Could you check a few things on this model? Use its own coordinates, in mm. A direction names the side the tool comes from. Round coordinates to 2 decimals unless told otherwise and drop trailing zeros. Order: outer loops, then holes, each group sorted by start corner. A loop starts at its lowest first (then second) coordinate and runs counter-clockwise, first axis right, second up. Notation, with made-up numbers: (18, 17) - (36, 17) arc R16 cw to (36, 25) - close; hole circle Ø3 at (50, 25). An arc over 180 degrees is marked (long way). Use one line per item in the form item = value.
from build123d import *

# Parameters (mm, degrees)
F1_DEPTH = 496
F2_R     = 6
F3_DEPTH = 40
F5_W     = 650
F5_H     = 10
F6_DEPTH = 10
F7_W     = 10
F7_H     = 476
F8_DEPTH = 10


# Not quite as in the source:
# - a pattern or mirror of a feature is missing from the dataset's text; its kind, count and spacing are read off the source's solid


with BuildPart() as f1:
    # F0 (on Front) → F1 (new body)
    with BuildSketch(Plane.XZ):
        Polygon((374.2424272732, 0), (-325.7575727268, 0), (-325.7575727268, -40), (-285.7575727268, -40), (-285.7575727268, -20), (344.2424272732, -20), (344.2424272732, -40), (374.2424272732, -40), align=None)
    extrude(amount=F1_DEPTH)

    # F2 (on face) → F3 (join)
    with BuildSketch(Plane(origin=(0, 0, 0), x_dir=(-1, 0, 0), z_dir=(0, 1, 0))):
        with Locations((-359.2424272732, -20)):
            Circle(F2_R)
        with Locations((305.7575727268, -20)):
            Circle(F2_R)
    f3 = extrude(amount=F3_DEPTH)

    # F3_copies: F3 across plane
    add(f3.mirror(Plane(origin=(0, -248, 0), x_dir=(0, 0, -1), z_dir=(0, -1, 0))))

    # F5 (on face) → F6 (cut)
    with BuildSketch(Plane(origin=(0, 0, 0), x_dir=(-1, 0, 0), z_dir=(0, 1, 0))):
        with Locations((-39.2424272732, -5)):
            Rectangle(F5_W, F5_H)
    f6 = extrude(amount=-F6_DEPTH, mode=Mode.SUBTRACT)

    # F6_copies: F6 across plane
    add(f6.mirror(Plane(origin=(0, -248, 0), x_dir=(0, 0, -1), z_dir=(0, -1, 0))), mode=Mode.SUBTRACT)

    # F7 (on face) → F8 (cut)
    with BuildSketch(Plane.XY):
        with Locations((359.2424272732, -248)):
            Rectangle(F7_W, F7_H)
    extrude(amount=-F8_DEPTH, mode=Mode.SUBTRACT)


solid = f1.part
Item 1: I need wall thicknesses on L1, parallel to X at y = -164.5, z = -33; L2, parallel to X at y = -142.5, z = -5.5; L3, parallel to Z at x = -101, y = -435.5. Which ranges of each line are inside material? Lowest first, please.
Found:
L1 = -325.76 to -285.76, 344.24 to 374.24
L2 = -325.76 to 354.24, 364.24 to 374.24
L3 = -20 to 0
Item 2: If we mould it in two halves opening along X, with no side actions, what happens to faces 1 (the face through (19, -245, 0)), 2 (the face through (374.242, -245, -20)), 3 (the face through (-58, -496, -15))? For each: released by +X, released by -X, zero draft, split by the parting line, or undercut.
Found:
face_1 = zero draft
face_2 = released by +X
face_3 = undercut
Item 3: Imagine slicing it at B-B on x = -8. Please give me the cut outline in (y, z).
Found:
outline = (-496, -20) - (0, -20) - (0, -10) - (-10, -10) - (-10, 0) - (-486, 0) - (-486, -10) - (-496, -10) - close
Item 4: Will these pins go through, and if not, where does the flat tip stop? P1, Ø3, axis at x = 144, z = -9, coming from the -Y side; P2, Ø5, axis at x = 14.5, z = -6.5, coming from the -Y side; P3, Ø2, axis at x = -13, z = -20, coming from the +Y side.
Found:
P1 = -496
P2 = -486
P3 = 0
Item 5: Imagine slicing it at A-A on y = -214.5. Please give me the cut outline in (x, z), plus the area to 3 significant figures.
Found:
outline = (-325.76, -40) - (-285.76, -40) - (-285.76, -20) - (344.24, -20) - (344.24, -40) - (374.24, -40) - (374.24, 0) - (364.24, 0) - (364.24, -10) - (354.24, -10) - (354.24, 0) - (-325.76, 0) - close
area = 15,300 mm2
Item 6: For faces 4 (the face through (-285.758, -245, -30)), 5 (the face through (-325.758, -245, -20)), which set-ups out of +Z, -Z, +X, -X, +Y, -Y let a thin tool reach every point of the face, with its end or its side?
Found:
face_4 = -Z, +Y, -Y
face_5 = +Z, -Z, -X, +Y, -Y
